from build123d import *

# Parameters (mm, degrees)
F0_W     = 26
F0_H     = 40
F1_DEPTH = 2
F2_W     = 30
F2_H     = 40
F3_DEPTH = 2
F4_W     = 2
F4_H     = 2
F4_H_2   = 2.5
F4_W_2   = 30
F4_W_3   = 22
F4_H_3   = 8
F4_H_4   = 29.5
F5_DEPTH = 2
F6_R     = 0.99999


# Not quite as in the source:
# - a fillet or chamfer is up to 0.001 mm smaller than in the source, because OpenCascade refuses the exact size


with BuildPart() as f1:
    # F0 (on Front) → F1 (new body)
    with BuildSketch(Plane.XZ):
        with Locations((-0.059209764, 5.0314570961)):
            Rectangle(F0_W, F0_H)
    extrude(amount=F1_DEPTH)

    # F2 (on face) → F3 (join)
    with BuildSketch(Plane.XZ.offset(2)):
        with Locations((-0.059209764, 5.0314570961)):
            Rectangle(F2_W, F2_H)
    extrude(amount=F3_DEPTH)

    # F4 (on face) → F5 (cut)
    with BuildSketch(Plane.XZ.offset(4)):
        with Locations((-14.059209764, 24.0314570961)):
            Rectangle(F4_W, F4_H)
        with Locations((13.940790236, 24.0314570961)):
            Rectangle(F4_W, F4_H)
        with Locations((-14.059209764, 19.7814570961)):
            Rectangle(F4_W, F4_H_2)
        with Locations((13.940790236, 19.7814570961)):
            Rectangle(F4_W, F4_H_2)
        with Locations((-0.059209764, -13.9685429039)):
            Rectangle(F4_W_2, F4_H)
        with Locations((-0.059209764, 21.7814570961)):
            Rectangle(F4_W_3, F4_H_2)
        with Locations((-14.059209764, 4.0314570961)):
            Rectangle(F4_W, F4_H_3)
        with Locations((13.940790236, 4.0314570961)):
            Rectangle(F4_W, F4_H_3)
        with Locations((-0.059209764, 3.7814570961)):
            Rectangle(F4_W_3, F4_H_4)
    extrude(amount=-F5_DEPTH, mode=Mode.SUBTRACT)

    # F6 (radius 1 in the source; OpenCascade refuses exactly that, so slightly less here)
    f6_edges = [f1.edges().sort_by_distance(p)[0] for p in [
        (14.94079, -3, 23.031457),
        (14.94079, -3, 21.031457),
        (14.94079, -3, 18.531457),
        (14.94079, -3, -12.968543),
        (-15.05921, -3, -12.968543),
        (-15.05921, -3, 18.531457),
        (-15.05921, -3, 23.031457),
        (-15.05921, -3, 21.031457),
        (-15.05921, -3, 8.031457),
        (-15.05921, -3, 0.031457),
        (14.94079, -3, 8.031457),
        (14.94079, -3, 0.031457),
        (-0.05921, -2, -10.968543),
        (10.94079, -2, 3.781457),
        (-0.05921, -2, 18.531457),
        (-11.05921, -2, 3.781457),
        (-0.05921, -4, 18.531457),
        (-11.05921, -4, 3.781457),
        (-0.05921, -4, -10.968543),
        (10.94079, -4, 3.781457),
    ]]
    fillet(f6_edges, radius=F6_R)


solid = f1.part
Check sheet for the modelled part. Datum: model origin and axes. Units: mm. A direction names the side the tool comes from. Round coordinates to 2 decimals unless told otherwise and drop trailing zeros. Loops run counter-clockwise (first coordinate to the right, second up) from the corner with the lowest first, then second, coordinate; pieces in that order, holes last. Notation, with made-up numbers: (-12, -15) -> (19, -15) arc R20 cw to (19, 18) -> close; hole circle Ø2 at (59.25, -35). An arc over 180 degrees is marked (long way). Put each result on its own line as item: value. Start each with the question number.
1. Access from +Z, -Z, +X, -X, +Y, -Y to the whole of each face (thin tool, end or side, straight path). Record for faces 1 (the face through (-13.6, -3, 23.031)), 2 (the face through (-14, -2, 22)), 3 (the face through (-11.36, -3.715, 4.002)).
2. Gauge pin test, flat ends, axial feed: pin 1 (16 mm diameter, centred on x = -1.5, z = 8.5, fed in from -Y); pin 2 (0.5 mm diameter, centred on x = 13.5, y = -2.5, fed in from +Z); pin 3 (10 mm diameter, centred on x = 9.5, z = 9.5, fed in from +Y); pin 4 (1 mm diameter, centred on x = 13.5, z = -4.5, fed in from +Y). Record the tip position at first contact, or that the pin passes through.
3. Section check C-C (y = -0.7). Enter the section's corners in (x, z), plus the area to 3 significant figures.
4. Draft check along X on faces 4 (the face through (14.64, -2.986, 21.317)), 5 (the face through (14, -2, 22)), 6 (the face through (-11.059, -3, 22)). Enter one of: +X half, -X half, draft (parallel to the pull), parting line (faces both ways), or undercut.
5. Scan lines: probe 1 along Z at (x, y) = (13, -2.05); probe 2 along Z at (x, y) = (3, -2.1); probe 3 along Y at (x, z) = (-1.5, -6). Record each from-to range of solid material in increasing order.
Findings:
1. face 1: +Z, -X, +Y, -Y
1. face 2: +Z, -Z, -X, +Y
1. face 3: -Y
2. pin 1: stops at y = -2
2. pin 2: stops at z = 23.03
2. pin 3: stops at y = 0
2. pin 4: stops at y = -2
3. outline: (-13.06, -14.97) -> (12.94, -14.97) -> (12.94, 25.03) -> (-13.06, 25.03) -> close
3. area: 1,040 mm^2
4. face 4: +X half
4. face 5: draft
4. face 6: undercut
5. probe 1: z = -12.97 to 0.03, 8.03 to 18.53, 21.03 to 23.03
5. probe 2: z = -12.97 to -10.4, 17.97 to 20.53, 23.03 to 25.03
5. probe 3: y = -2 to 0
